Build history of the part. All positions in model axes, mm. Face numbers are marked on the shaded views. A direction names the side the tool comes from. Give positions to 0.01 mm unless a question says otherwise; leave off trailing zeros. Loops run counter-clockwise (first coordinate to the right, second up) from the corner with the lowest first, then second, coordinate; pieces in that order, holes last. Notation, with made-up numbers: M -0.75,-38.75 L 58.25,-38.75 A16 ccw 58.25,-30.75 Z; hole C 58.25,-11 d2. An arc over 180 degrees is marked long. Answer in a Markdown table with one row per item. Add a question column.
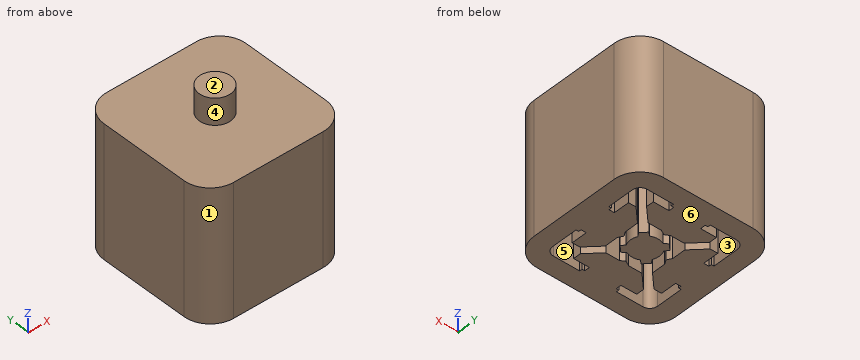
```python
from build123d import *

# Parameters (mm, degrees)
BOSS_EXTRU_5_DEPTH = 15
BOSS_EXTRU_6_DEPTH = 10
ESQUISSE7_R        = 3
BOSS_EXTRU_7_DEPTH = 5


# Read off the part's stored shape, not the designer's step: Boss.-Extru.5
with BuildPart() as part:
    # Boss.-Extru.5 outline → Boss.-Extru.5 (new body)
    # profile 1 of 2: a face of its own
    with BuildSketch(Plane.XY):
        with BuildLine():
            Line((-8.5, -13.5), (8.5, -13.5))
            ThreePointArc((8.5, -13.5), (12.035533906, -12.035533906), (13.5, -8.5))
            Line((13.5, -8.5), (13.5, 8.5))
            ThreePointArc((13.5, 8.5), (12.035533906, 12.035533906), (8.5, 13.5))
            Line((8.5, 13.5), (-8.5, 13.5))
            ThreePointArc((-8.5, 13.5), (-12.035533906, 12.035533906), (-13.5, 8.5))
            Line((-13.5, 8.5), (-13.5, -8.5))
            ThreePointArc((-13.5, -8.5), (-12.035533906, -12.035533906), (-8.5, -13.5))
        make_face()
        with BuildLine():
            Line((-10, 3.5), (-10, 8.5))
            ThreePointArc((-10, 8.5), (-9.560660172, 9.560660172), (-8.5, 10))
            Line((-8.5, 10), (-3.5, 10))
            Line((-3.5, 10), (-3.5, 9.5))
            Line((-3.5, 9.5), (-3, 9.5))
            Line((-3, 9.5), (-3, 8.5))
            Line((-3, 8.5), (-6, 8.5))
            Line((-6, 8.5), (-6, 7.060660172))
            Line((-6, 7.060660172), (-3.439339828, 4.5))
            Line((-3.439339828, 4.5), (-0.866025404, 4.5))
            Line((-0.866025404, 4.5), (0, 4))
            Line((0, 4), (0.866025404, 4.5))
            Line((0.866025404, 4.5), (3.439339828, 4.5))
            Line((3.439339828, 4.5), (6, 7.060660172))
            Line((6, 7.060660172), (6, 8.5))
            Line((6, 8.5), (3, 8.5))
            Line((3, 8.5), (3, 9.5))
            Line((3, 9.5), (3.5, 9.5))
            Line((3.5, 9.5), (3.5, 10))
            Line((3.5, 10), (8.5, 10))
            ThreePointArc((8.5, 10), (9.560660172, 9.560660172), (10, 8.5))
            Line((10, 8.5), (10, 3.5))
            Line((10, 3.5), (9.5, 3.5))
            Line((9.5, 3.5), (9.5, 3))
            Line((9.5, 3), (8.5, 3))
            Line((8.5, 3), (8.5, 6))
            Line((8.5, 6), (7.060660172, 6))
            Line((7.060660172, 6), (4.5, 3.439339828))
            Line((4.5, 3.439339828), (4.5, 0.866025404))
            Line((4.5, 0.866025404), (4, 0))
            Line((4, 0), (4.5, -0.866025404))
            Line((4.5, -0.866025404), (4.5, -3.439339828))
            Line((4.5, -3.439339828), (7.060660172, -6))
            Line((7.060660172, -6), (8.5, -6))
            Line((8.5, -6), (8.5, -3))
            Line((8.5, -3), (9.5, -3))
            Line((9.5, -3), (9.5, -3.5))
            Line((9.5, -3.5), (10, -3.5))
            Line((10, -3.5), (10, -8.5))
            ThreePointArc((10, -8.5), (9.560660172, -9.560660172), (8.5, -10))
            Line((8.5, -10), (3.5, -10))
            Line((3.5, -10), (3.5, -9.5))
            Line((3.5, -9.5), (3, -9.5))
            Line((3, -9.5), (3, -8.5))
            Line((3, -8.5), (6, -8.5))
            Line((6, -8.5), (6, -7.060660172))
            Line((6, -7.060660172), (3.439339828, -4.5))
            Line((3.439339828, -4.5), (0.866025404, -4.5))
            Line((0.866025404, -4.5), (0, -4))
            Line((0, -4), (-0.866025404, -4.5))
            Line((-0.866025404, -4.5), (-3.439339828, -4.5))
            Line((-3.439339828, -4.5), (-6, -7.060660172))
            Line((-6, -7.060660172), (-6, -8.5))
            Line((-6, -8.5), (-3, -8.5))
            Line((-3, -8.5), (-3, -9.5))
            Line((-3, -9.5), (-3.5, -9.5))
            Line((-3.5, -9.5), (-3.5, -10))
            Line((-3.5, -10), (-8.5, -10))
            ThreePointArc((-8.5, -10), (-9.560660172, -9.560660172), (-10, -8.5))
            Line((-10, -8.5), (-10, -3.5))
            Line((-10, -3.5), (-9.5, -3.5))
            Line((-9.5, -3.5), (-9.5, -3))
            Line((-9.5, -3), (-8.5, -3))
            Line((-8.5, -3), (-8.5, -6))
            Line((-8.5, -6), (-7.060660172, -6))
            Line((-7.060660172, -6), (-4.5, -3.439339828))
            Line((-4.5, -3.439339828), (-4.5, -0.866025404))
            Line((-4.5, -0.866025404), (-4, 0))
            Line((-4, 0), (-4.5, 0.866025404))
            Line((-4.5, 0.866025404), (-4.5, 3.439339828))
            Line((-4.5, 3.439339828), (-7.060660172, 6))
            Line((-7.060660172, 6), (-8.5, 6))
            Line((-8.5, 6), (-8.5, 3))
            Line((-8.5, 3), (-9.5, 3))
            Line((-9.5, 3), (-9.5, 3.5))
            Line((-9.5, 3.5), (-10, 3.5))
        make_face(mode=Mode.SUBTRACT)
    # profile 2 of 2: a face of its own
    with BuildSketch(Plane.XY):
        with BuildLine():
            Line((1.949592103, 3.000876196), (1.276279893, 2.435900169))
            ThreePointArc((1.276279893, 2.435900169), (0.001756003, 2.749999439), (-1.273167982, 2.43752811))
            Line((-1.273167982, 2.43752811), (-1.947287092, 3.003181207))
            Line((-1.947287092, 3.003181207), (-3.000876196, 1.949592103))
            Line((-3.000876196, 1.949592103), (-2.435900169, 1.276279893))
            ThreePointArc((-2.435900169, 1.276279893), (-2.749999439, 0.001756003), (-2.43752811, -1.273167982))
            Line((-2.43752811, -1.273167982), (-3.003181207, -1.947287092))
            Line((-3.003181207, -1.947287092), (-1.949592103, -3.000876196))
            Line((-1.949592103, -3.000876196), (-1.276279893, -2.435900169))
            ThreePointArc((-1.276279893, -2.435900169), (-0.001756003, -2.749999439), (1.273167982, -2.43752811))
            Line((1.273167982, -2.43752811), (1.947287092, -3.003181207))
            Line((1.947287092, -3.003181207), (3.000876196, -1.949592103))
            Line((3.000876196, -1.949592103), (2.435900169, -1.276279893))
            ThreePointArc((2.435900169, -1.276279893), (2.749999439, -0.001756003), (2.43752811, 1.273167982))
            Line((2.43752811, 1.273167982), (3.003181207, 1.947287092))
            Line((3.003181207, 1.947287092), (1.949592103, 3.000876196))
        make_face()
    extrude(amount=BOSS_EXTRU_5_DEPTH)

    # Esquisse6 → Boss.-Extru.6 (add)
    with BuildSketch(Plane.XY.offset(15)):
        with BuildLine():
            Line((-13.5, 8.5), (-13.5, -8.5))
            ThreePointArc((-13.5, -8.5), (-12.035533906, -12.035533906), (-8.5, -13.5))
            Line((-8.5, -13.5), (8.5, -13.5))
            ThreePointArc((8.5, -13.5), (12.035533906, -12.035533906), (13.5, -8.5))
            Line((13.5, -8.5), (13.5, 8.5))
            ThreePointArc((13.5, 8.5), (12.035533906, 12.035533906), (8.5, 13.5))
            Line((8.5, 13.5), (-8.5, 13.5))
            ThreePointArc((-8.5, 13.5), (-12.035533906, 12.035533906), (-13.5, 8.5))
        make_face()
    extrude(amount=BOSS_EXTRU_6_DEPTH)

    # Esquisse7 → Boss.-Extru.7 (add)
    with BuildSketch(Plane.XY.offset(25)):
        Circle(ESQUISSE7_R)
    extrude(amount=BOSS_EXTRU_7_DEPTH)


solid = part.part
```
(1) Pull direction Y, two halves, no side cores. Call the marked faces 1, 2 and 3: +Y half, -Y half, draft (parallel to the pull), parting line (faces both ways), or undercut.
(2) Slice it at C-C, the plane y = -11.5. Give the cut face in (x, z), then the cut area to 3 significant figures.
(3) Wall check: line 1 (Y direction, x = 0, z = 11.75); line 2 (Y direction, x = 1, z = 12); line 3 (X direction, y = 8, z = 4.25). Give the ranges that are in metal, low to high.
(4) Slice it at D-D, the plane y = 9. Give the cut face in (x, z).
(5) Pin check, flat tips, straight feed: pin 1 (0.5 mm diameter, centred on y = -9, z = 9.5, fed in from +X); pin 2 (6 mm diameter, centred on x = -6.5, y = -8, fed in from +Z). Stop position of each tip, or through.
(6) Slice it at B-B, the plane z = 7.5. State how many separate pieces and enclosed holes the cut face has, then the cut area to 3 significant figures.
(7) Tool access for the marked faces 4, 5 and 6: list every direction of +Z, -Z, +X, -X, +Y, -Y with a clear straight run to the whole face (end or side of a thin tool).
(8) Slice it at A-A, the plane x = -7.75. Give the cut face in (y, z), then the cut area to 3 significant figures.
Solution:
| question | item | result |
|---|---|---|
| 1 | face 1 | -Y half |
| 1 | face 2 | draft |
| 1 | face 3 | undercut |
| 2 | outline | M -12.5,0 L 12.5,0 L 12.5,25 L -12.5,25 Z |
| 2 | area | 625 mm^2 |
| 3 | line 1 | -13.5 to -4, -2.75 to 2.75, 4 to 13.5 |
| 3 | line 2 | -13.5 to -4.5, -2.56 to 2.56, 4.5 to 13.5 |
| 3 | line 3 | -13.5 to -10, -6 to 6, 10 to 13.5 |
| 4 | outline | M -13.47,0 L -9.91,0 L -9.91,15 L -3,15 L -3,0 L 3,0 L 3,15 L 9.91,15 L 9.91,0 L 13.47,0 L 13.47,25 L -13.47,25 Z |
| 5 | pin 1 | x = 13.49 |
| 5 | pin 2 | z = 25 |
| 6 | separate pieces | 2 |
| 6 | enclosed holes | 1 |
| 6 | area | 544 mm^2 |
| 7 | face 4 | +Z |
| 7 | face 5 | -Z |
| 7 | face 6 | -Z, +X, -X, +Y, -Y |
| 8 | outline | M -13.5,0 L -10,0 L -10,15 L -6,15 L -6,0 L 6,0 L 6,15 L 10,15 L 10,0 L 13.5,0 L 13.5,25 L -13.5,25 Z |
| 8 | area | 555 mm^2 |
